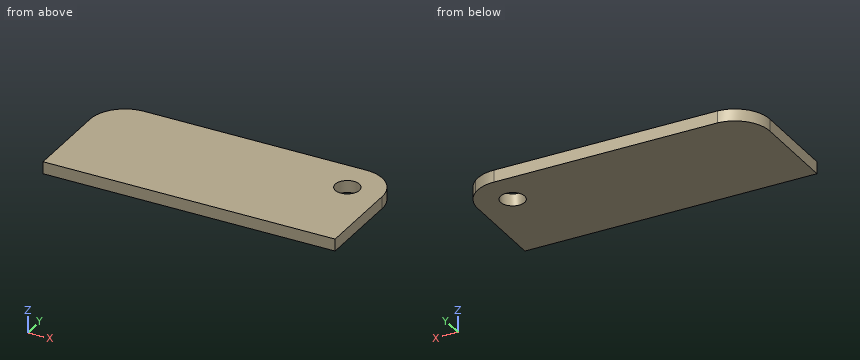
from build123d import *

# Parameters (mm, degrees)
SKETCH1_W           = 6.477
SKETCH1_H           = 19.812
SKETCH1_R           = 1.5
SKETCH1_W_2         = 52.832
SKETCH1_H_2         = 5
BOSS_EXTRUDE2_DEPTH = 3.175
SKETCH3_W           = 30
SKETCH3_H           = 29.812
BOSS_EXTRUDE3_DEPTH = 3.175
SKETCH4_R           = 3.175
CUT_EXTRUDE1_DEPTH  = 10
SKETCH5_W           = 56.703294506
SKETCH5_H           = 29.812
BOSS_EXTRUDE4_DEPTH = 3.175
BOSS_EXTRUDE6_DEPTH = 3.175
CUT_EXTRUDE3_DEPTH  = 10
SKETCH11_R          = 3.175
BOSS_EXTRUDE7_DEPTH = 3.175
CUT_EXTRUDE4_START  = -3.175
CUT_EXTRUDE4_DEPTH  = 3.175
SKETCH13_R          = 3.175
BOSS_EXTRUDE8_DEPTH = 3.175


# Read off the part's stored shape, not the designer's step: Cut-Extrude4
with BuildPart() as part:
    # Sketch1 → Boss-Extrude2 (new body)
    # profile 1 of 4: a face of its own
    with BuildSketch(Plane.XY):
        with Locations((-23.1775, 0)):
            Rectangle(SKETCH1_W, SKETCH1_H)
        with Locations((-23.622, -5.08)):
            Circle(SKETCH1_R, mode=Mode.SUBTRACT)
        with Locations((-23.622, 5.08)):
            Circle(SKETCH1_R, mode=Mode.SUBTRACT)
    # profile 2 of 4: a face of its own
    with BuildSketch(Plane.XY):
        with Locations((23.1775, 0)):
            Rectangle(SKETCH1_W, SKETCH1_H)
        with Locations((23.622, -5.08)):
            Circle(SKETCH1_R, mode=Mode.SUBTRACT)
        with Locations((23.622, 5.08)):
            Circle(SKETCH1_R, mode=Mode.SUBTRACT)
    # profile 3 of 4: a face of its own
    with BuildSketch(Plane.XY):
        with Locations((0, 12.406)):
            Rectangle(SKETCH1_W_2, SKETCH1_H_2)
    # profile 4 of 4: a face of its own
    with BuildSketch(Plane.XY):
        with Locations((0, -12.406)):
            Rectangle(SKETCH1_W_2, SKETCH1_H_2)
    extrude(amount=BOSS_EXTRUDE2_DEPTH)

    # Sketch3 → Boss-Extrude3 (add)
    with BuildSketch(Plane.XY.offset(3.175)):
        with Locations((41.416, 0)):
            Rectangle(SKETCH3_W, SKETCH3_H)
    extrude(amount=-BOSS_EXTRUDE3_DEPTH)

    # Sketch4 → Cut-Extrude1 (cut)
    with BuildSketch(Plane(origin=(0, 0, 0), x_dir=(-1, 0, 0), z_dir=(0, 0, -1))):
        with Locations((-41.266, 8.006)):
            Circle(SKETCH4_R)
    extrude(amount=-CUT_EXTRUDE1_DEPTH, mode=Mode.SUBTRACT)

    # Sketch5 → Boss-Extrude4 (add)
    with BuildSketch(Plane(origin=(0, 0, 0), x_dir=(-1, 0, 0), z_dir=(0, 0, -1))):
        with Locations((-1.935647253, 0)):
            Rectangle(SKETCH5_W, SKETCH5_H)
    extrude(amount=-BOSS_EXTRUDE4_DEPTH)

    # Sketch8 → Boss-Extrude6 (add)
    with BuildSketch(Plane(origin=(0, 0, 0), x_dir=(-1, 0, 0), z_dir=(0, 0, -1))):
        with BuildLine():
            ThreePointArc((-21.596379237, 14.906), (-31.366874619, 16.599566662), (-41.266, 17.181))
            ThreePointArc((-41.266, 17.181), (-44.496566901, 16.593436317), (-47.313365129, 14.906))
            Line((-47.313365129, 14.906), (-21.596379237, 14.906))
        make_face()
    extrude(amount=-BOSS_EXTRUDE6_DEPTH)

    # Sketch9 → Cut-Extrude3 (cut)
    with BuildSketch(Plane(origin=(0, 0, 0), x_dir=(-1, 0, 0), z_dir=(0, 0, -1))):
        with BuildLine():
            Line((-50.441, -14.906), (-50.441, 8.006))
            ThreePointArc((-50.441, 8.006), (-49.622590215, 11.79387869), (-47.313365129, 14.906))
            Line((-47.313365129, 14.906), (-56.416, 14.906))
            Line((-56.416, 14.906), (-56.416, -14.906))
            Line((-56.416, -14.906), (-50.441, -14.906))
        make_face()
        with BuildLine():
            ThreePointArc((-21.596379237, 14.906), (4.87312141, 3.967175073), (26.416, -14.906))
            Line((26.416, -14.906), (26.416, 14.906))
            Line((26.416, 14.906), (-21.596379237, 14.906))
        make_face()
    extrude(amount=-CUT_EXTRUDE3_DEPTH, mode=Mode.SUBTRACT)

    # Sketch11 → Boss-Extrude7 (add)
    with BuildSketch(Plane(origin=(0, 0, 0), x_dir=(-1, 0, 0), z_dir=(0, 0, -1))):
        with BuildLine():
            ThreePointArc((-41.266, 17.181), (-3.83303759, 8.714126043), (26.416, -14.906))
            Line((26.416, -14.906), (26.416, 17.181))
            Line((26.416, 17.181), (-41.266, 17.181))
        make_face()
        with Locations((17.236, 8.006)):
            Circle(SKETCH11_R, mode=Mode.SUBTRACT)
    extrude(amount=-BOSS_EXTRUDE7_DEPTH)

    # Cut-Extrude4 outline → Cut-Extrude4 (cut)
    with BuildSketch(Plane(origin=(0, 0, 0), x_dir=(-1, 0, 0), z_dir=(0, 0, -1)).offset(CUT_EXTRUDE4_START)):
        with BuildLine():
            ThreePointArc((17.538943889, 17.181), (23.833477734, 14.389234881), (26.416, 8.006))
            Line((26.416, 8.006), (26.416, 17.181))
            Line((26.416, 17.181), (17.538943889, 17.181))
        make_face()
    extrude(amount=CUT_EXTRUDE4_DEPTH, mode=Mode.SUBTRACT)

    # Sketch13 → Boss-Extrude8 (add)
    with BuildSketch(Plane(origin=(0, 0, 0), x_dir=(-1, 0, 0), z_dir=(0, 0, -1))):
        with Locations((17.236, 8.006)):
            Circle(SKETCH13_R)
    extrude(amount=-BOSS_EXTRUDE8_DEPTH)


solid = part.part
Here's how the part is built. I have some questions about the finished solid (model axes, mm). Coordinates: 2 decimals unless noted, no trailing zeros. Write each loop counter-clockwise with the first axis right and the second up, starting at its lowest first coordinate (ties: lowest second). Pieces come first, ordered by that corner, then holes.
Item 1: I want a section at A-A on z = 1.8. Write out the boundary of the cut face in (x, y) (3 decimals).
Item 2: Will these pins go through, and if not, where does the flat tip stop? pin 1 (1.5 mm diameter, centred on y = 13.5, z = 2, fed in from -X); pin 2 (6 mm diameter, centred on x = 38.5, y = -10.5, fed in from -Z); pin 3 (4 mm diameter, centred on x = 41.266, y = 8.006, fed in from -Z).
Item 3: I want a section at B-B on y = 6. Write out the boundary of the cut face in (x, z) (3 decimals).
Item 4: I want a section at C-C on x = -21. Write out the boundary of the cut face in (y, z) (3 decimals), and give its area (3 significant figures).
Item 5: If I drill on line 1 (X direction, y = 8, z = 2.3); line 2 (X direction, y = 10, z = 1.6); line 3 (Y direction, x = -20, z = 2.05), over which ranges is the centre line in solid material (lowest first)?
Findings below:
1. outline: (-26.416, -14.906) - (50.441, -14.906) - (50.441, 8.006) arc R9.175 ccw to (41.266, 17.181) - (-17.539, 17.181) arc R9.18 ccw to (-26.416, 8.006) - close; hole circle Ø6.35 at (41.266, 8.006)
2. pin 1: stops at x = -25.1
2. pin 2: stops at z = 0
2. pin 3: passes through
3. outline: (-26.416, 0) - (38.805, 0) - (38.805, 3.175) - (-26.416, 3.175) - close; (43.727, 0) - (50.441, 0) - (50.441, 3.175) - (43.727, 3.175) - close
4. outline: (-14.906, 0) - (16.379, 0) - (16.379, 3.175) - (-14.906, 3.175) - close
4. area: 99.3 mm2
5. line 1: x = -26.42 to 38.09, 44.44 to 50.44
5. line 2: x = -26.2 to 38.8, 43.74 to 50.22
5. line 3: y = -14.91 to 16.76
